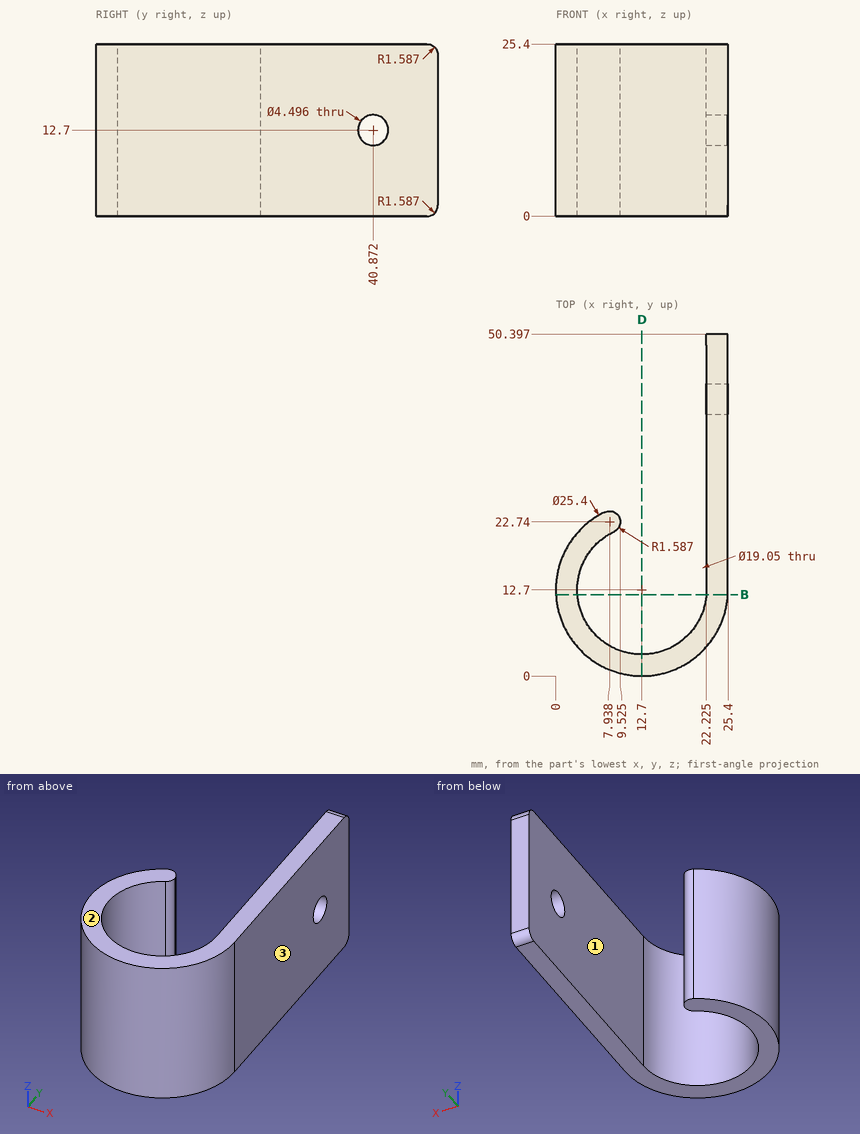
Can you work these out from the drawing? Everything is in mm from the part's minimum corner. Coordinates: 2 decimals unless noted, no trailing zeros. Order: outer loops, then holes, each group sorted by start corner. A loop starts at its lowest first (then second) coordinate and runs counter-clockwise, first axis right, second up. Notation, with made-up numbers: M 35,53.25 L 91,53.25 A30 cw 91,79.25 Z; hole C 11.25,74 d7. An arc over 180 degrees is marked long. Answer as CSV lines item,"result". Start each with the question number.
1. For pin 1 (10 mm diameter, centred on x = 4, y = 31, fed in from -Z); pin 2 (10 mm diameter, centred on x = 14, z = 7, fed in from +Y); pin 3 (3 mm diameter, centred on x = 17.5, z = 22.5, fed in from -Y); pin 4 (1 mm diameter, centred on y = 41.5, z = 10, fed in from -X) (1 decimal), each with a flat end and sliding along its axis, tell me the tip position at first contact or that it passes through.
2. We'd pull the mould along X, two halves only. Please class the marked faces 1, 2 and 3: released by +X, released by -X, zero draft, split by the parting line, or undercut.
3. I want a section at B-B, the plane y = 12. Write out the boundary of the cut face in (x, z).
4. I need wall thicknesses on line 1 (X direction, y = 12.7, z = 10) (1 decimal); line 2 (Y direction, x = 12.7, z = 9.75) (1 decimal); line 3 (X direction, y = 39, z = 15.75) (1 decimal). Which ranges of each line are inside material? Lowest first, please. Write a range as [from, to].
5. I want a section at D-D, the plane x = 12.7. Write out the boundary of the cut face in (y, z) (1 decimal).
Recorded:
1,pin 1,"passes through"
1,pin 2,"stops at y = 23.92"
1,pin 3,"stops at y = 0.44"
1,pin 4,"stops at x = 22.2"
2,face 1,"undercut"
2,face 2,"zero draft"
2,face 3,"released by +X"
3,outline,"M 0.02,0 L 3.2,0 L 3.2,25.4 L 0.02,25.4 Z; M 22.2,0 L 25.38,0 L 25.38,25.4 L 22.2,25.4 Z"
4,line 1,"x = [0, 3.2], [22.2, 25.4]"
4,line 2,"y = [0, 3.2]"
4,line 3,"x = [22.2, 25.4]"
5,outline,"M 0,0 L 3.2,0 L 3.2,25.4 L 0,25.4 Z"
